Check sheet for the drawn part. Datum: minimum x, y, z corner. Units: mm. A direction names the side the tool comes from. Round coordinates to 2 decimals unless told otherwise and drop trailing zeros. Write each loop counter-clockwise with the first axis right and the second up, starting at its lowest first coordinate (ties: lowest second). Pieces come first, ordered by that corner, then holes. Notation, with made-up numbers: M 55,42 L 96,42 A17 cw 96,73 Z; hole C -11,0.25 d1. An arc over 180 degrees is marked long. One line per item, written item: value. Start each with the question number.
Item 1: Draft check along X on the marked faces 1, 2, 3 and 4. Enter one of: +X half, -X half, draft (parallel to the pull), parting line (faces both ways), or undercut.
Item 2: Tool access check on the marked faces 5 and 6. Record the directions out of +Z, -Z, +X, -X, +Y, -Y that give a thin tool (end or side, any length) a straight path to the whole face; none if there is none.
Item 3: Thickness scan on probe 1 along X at (y, z) = (9, 7); probe 2 along Z at (x, y) = (55.5, 15.5) (1 decimal); probe 3 along Y at (x, z) = (46, 20.5). Record the ranges inside material, lowest first. Write a range as from..to.
Item 4: Section check A-A, the plane y = 36.5. Record the cut outline in (x, z).
Item 5: Gauge pin test, flat ends, axial feed: pin 1 (11.5 mm diameter, centred on y = 16.002, z = 38.1, fed in from +X); pin 2 (4 mm diameter, centred on y = 48.5, z = 49.5, fed in from +X); pin 3 (1 mm diameter, centred on x = 36.5, z = 43.5, fed in from -Y). Record the tip position at first contact, or that the pin passes through.
Item 6: Section check C-C, the plane z = 15.24. Record the cut outline in (x, y), then the cut area to 3 significant figures.
Item 7: Section check B-B, the plane z = 38.1. State how many separate pieces and enclosed holes the cut face has, then the cut area to 3 significant figures.
Item 8: Section check D-D, the plane x = 33. Record the cut outline in (y, z) (1 decimal).
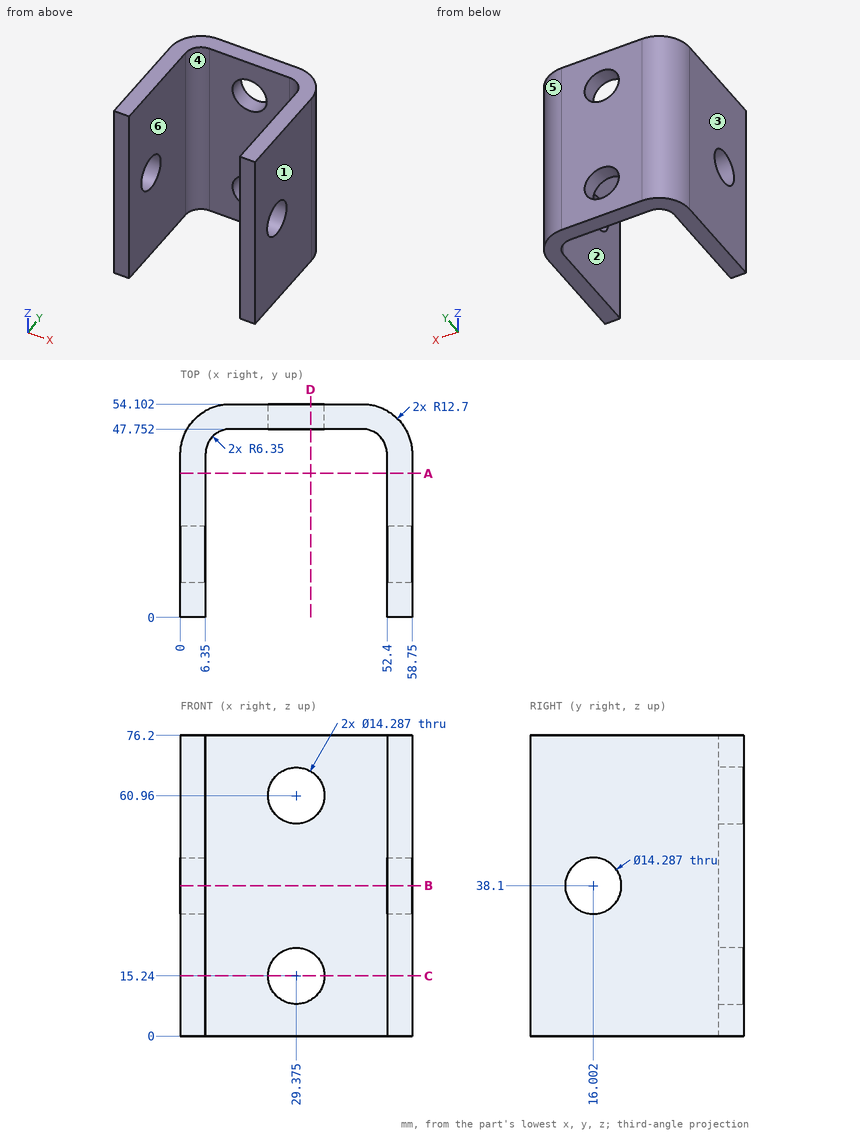
Response values:
1. face 1: +X half
1. face 2: undercut
1. face 3: -X half
1. face 4: undercut
2. face 5: +Z, -Z, +X, +Y
2. face 6: +Z, -Z, -Y
3. probe 1: x = 0..6.35, 52.4..58.75
3. probe 2: z = 0..31, 45.2..76.2
3. probe 3: y = 47.75..54.1
4. outline: M 0,0 L 6.35,0 L 6.35,76.2 L 0,76.2 Z; M 52.4,0 L 58.75,0 L 58.75,76.2 L 52.4,76.2 Z
5. pin 1: passes through
5. pin 2: stops at x = 57.68
5. pin 3: stops at y = 47.75
6. outline: M 0,0 L 6.35,0 L 6.35,41.4 A6.35 cw 12.7,47.75 L 22.23,47.75 L 22.23,54.1 L 12.7,54.1 A12.7 ccw 0,41.4 Z; M 36.52,47.75 L 46.05,47.75 A6.35 cw 52.4,41.4 L 52.4,0 L 58.75,0 L 58.75,41.4 A12.7 ccw 46.05,54.1 L 36.52,54.1 Z
6. area: 837 mm2
7. separate pieces: 3
7. enclosed holes: 0
7. area: 746 mm2
8. outline: M 47.8,0 L 54.1,0 L 54.1,9.1 L 47.8,9.1 Z; M 47.8,21.4 L 54.1,21.4 L 54.1,54.8 L 47.8,54.8 Z; M 47.8,67.1 L 54.1,67.1 L 54.1,76.2 L 47.8,76.2 Z
